Could you check a few things on this model? Use its own coordinates, in mm. Face numbers are marked on the shaded views. A direction names the side the tool comes from. Coordinates: 2 decimals unless noted, no trailing zeros. Write each loop counter-clockwise with the first axis right and the second up, starting at its lowest first coordinate (ties: lowest second). Pieces come first, ordered by that corner, then holes. Notation, with made-up numbers: (54, 46.25) - (68, 46.25) arc R20 cw to (68, 71.25) - close; hole circle Ø9 at (57.25, 75.5). An arc over 180 degrees is marked (long way). Answer as a JSON object with one key per item and string values. Group by question number.
1) Please list where these lines run through material, in increasing order: line 1 along Y through (x, z) = (28.5, 0.2); line 2 along Y through (x, z) = (0, 0.05); line 3 along X through (y, z) = (-2.5, -0.45).
2) Will these pins go through, and if not, where does the flat tip stop? pin 1 Ø1 at (y, z) = (-6, 0) entering from +X; pin 2 Ø1.2 at (x, z) = (21.5, 0) entering from +Y.
3) We'd pull the mould along X, two halves only. Please class the marked faces 5, 6, 7 and 8: released by +X, released by -X, zero draft, split by the parting line, or undercut.
4) On a 3-axis mill with a long thin cutter (end or side, diameter ignored), from which of +Z, -Z, +X, -X, +Y, -Y can I reach the whole of each face in a straight line? I mean the marked faces 1, 2, 3 and 4. Say none if no direction works.
5) If we section it at C-C (y = 0): Write out the boundary of the cut face in (x, z).
6) If we section it at B-B (z = 0.4): Write out the boundary of the cut face in (x, y).
7) If we section it at A-A (x = 25): Write out the boundary of the cut face in (y, z), plus the area to 3 significant figures.
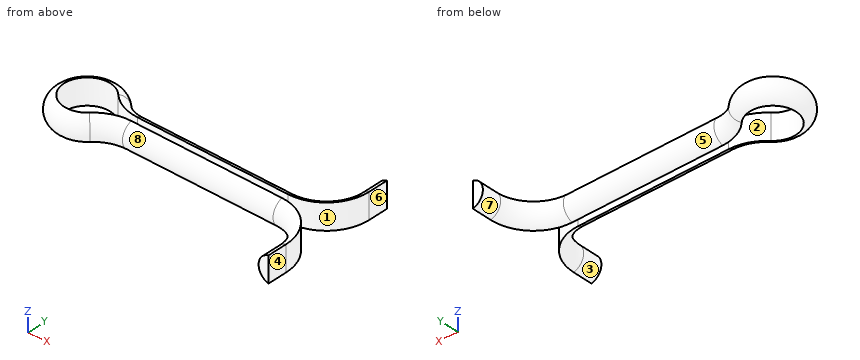
```python
from build123d import *


with BuildPart() as part:
    # Táhnout po křivce1: sweep along a path in Skica2
    with BuildLine(Plane.XY) as t_hnout_po_k_ivce1_path:
        Line((35, 10), (35, 7))
        ThreePointArc((35, 7), (33.535533906, 3.464466094), (30, 2))
        Line((30, 2), (7.141428429, 2))
        ThreePointArc((7.141428429, 2), (5.204936755, 2.390227771), (3.570714214, 3.5))
        ThreePointArc((3.570714214, 3.5), (-5, 0), (3.570714214, -3.5))
        ThreePointArc((3.570714214, -3.5), (5.204936755, -2.390227771), (7.141428429, -2))
        Line((7.141428429, -2), (30, -2))
        ThreePointArc((30, -2), (33.535533906, -3.464466094), (35, -7))
        Line((35, -7), (35, -10))
    # Skica4 → Táhnout po křivce1 (sweep)
    with BuildSketch(Plane(origin=(35, 10, 0), x_dir=(-1, 0, 0), z_dir=(0, -1, 0))):
        with BuildLine():
            Line((-1.5, 1.936491673), (-1.5, -1.936491673))
            ThreePointArc((-1.5, -1.936491673), (0, 0), (-1.5, 1.936491673))
        make_face()
    sweep(path=t_hnout_po_k_ivce1_path.line)


solid = part.part
```
Here are the results:
{
 "1": {"line 1": "y = -1.99 to -0.5, 0.5 to 1.99", "line 2": "y = -5 to -3.5, 3.5 to 5", "line 3": "x = -4.27 to -2.45, 2.45 to 4.85, 32.29 to 34.69"},
 "2": {"pin 1": "stops at x = 36.48", "pin 2": "stops at y = 2"},
 "3": {"face 5": "undercut", "face 6": "released by +X", "face 7": "released by -X", "face 8": "undercut"},
 "4": {"face 1": "+Z, -Z, +X", "face 2": "+Z, -Z", "face 3": "-X, -Y", "face 4": "+Z, -Z, +X, +Y, -Y"},
 "5": {"outline": "(-3.5, -1.94) - (-3.5, 1.94) arc R2 ccw to start"},
 "6": {"outline": "(2.5, -2.45) arc R3.5 cw (long way) to (2.5, 2.45) arc R6.5 ccw to (7.14, 0.5) - (30, 0.5) arc R6.5 ccw to (36.5, 7) - (36.5, 10) - (35.04, 10) - (35.04, 7) arc R5.04 cw to (30, 1.96) - (7.14, 1.96) arc R5.04 cw to (3.54, 3.47) arc R4.96 ccw (long way) to (3.54, -3.47) arc R5.04 cw to (7.14, -1.96) - (30, -1.96) arc R5.04 cw to (35.04, -7) - (35.04, -10) - (36.5, -10) - (36.5, -7) arc R6.5 ccw to (30, -0.5) - (7.14, -0.5) arc R6.5 ccw to start"},
 "7": {"outline": "(-0.5, -1.94) - (-0.5, 1.94) arc R2 ccw to start; (0.5, -1.94) arc R2 ccw to (0.5, 1.94) - close", "area": "8.61 mm²"}
}
